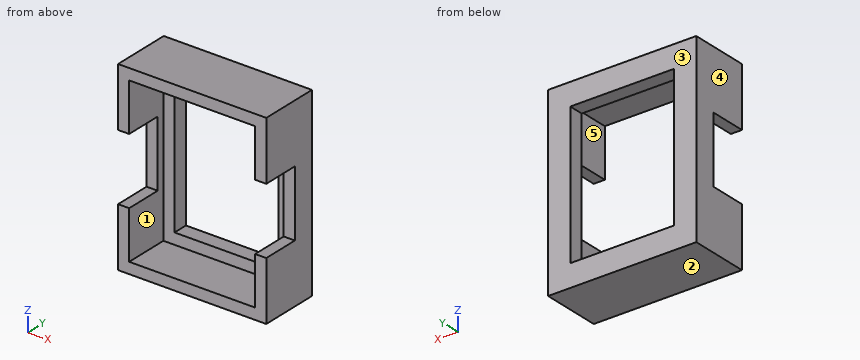
from build123d import *

# Parameters (mm, degrees)
SKETCH1_W           = 20
SKETCH1_H           = 25
BOSS_EXTRUDE1_DEPTH = 8
SKETCH2_W           = 9
SKETCH2_H           = 5
CUT_EXTRUDE1_DEPTH  = 31
SKETCH3_W           = 17
SKETCH3_H           = 22
CUT_EXTRUDE2_DEPTH  = 6
SKETCH4_W           = 14
SKETCH4_H           = 19
CUT_EXTRUDE3_DEPTH  = 7


with BuildPart() as part:
    # Sketch1 → Boss-Extrude1 (new body)
    with BuildSketch(Plane(origin=(0, 0, 0), x_dir=(1, 0, 0), z_dir=(0, 1, 0))):
        with Locations((-10.903225806, -2.629032258)):
            Rectangle(SKETCH1_W, SKETCH1_H)
    extrude(amount=BOSS_EXTRUDE1_DEPTH)

    # Sketch2 → Cut-Extrude1 (cut)
    with BuildSketch(Plane.ZY.offset(20.903225806)):
        with Locations((2.629032258, 2.5)):
            Rectangle(SKETCH2_W, SKETCH2_H)
    extrude(amount=-CUT_EXTRUDE1_DEPTH, mode=Mode.SUBTRACT)

    # Sketch3 → Cut-Extrude2 (cut)
    with BuildSketch(Plane.XZ):
        with Locations((-10.903225806, 2.629032258)):
            Rectangle(SKETCH3_W, SKETCH3_H)
    extrude(amount=-CUT_EXTRUDE2_DEPTH, mode=Mode.SUBTRACT)

    # Sketch4 → Cut-Extrude3 (cut)
    with BuildSketch(Plane(origin=(0, 8, 0), x_dir=(1, 0, 0), z_dir=(0, 1, 0))):
        with Locations((-10.903225806, -2.629032258)):
            Rectangle(SKETCH4_W, SKETCH4_H)
    extrude(amount=-CUT_EXTRUDE3_DEPTH, mode=Mode.SUBTRACT)


solid = part.part
Geometry check sheet. Reference: the model listing, model coordinates, mm. Face numbers are marked on the shaded views. A direction names the side the tool comes from. Coordinates: 2 decimals unless noted, no trailing zeros. Order: outer loops, then holes, each group sorted by start corner. A loop starts at its lowest first (then second) coordinate and runs counter-clockwise, first axis right, second up. Notation, with made-up numbers: (54.5, -24) - (88.5, -24) arc R21 cw to (88.5, 2) - close; hole circle Ø6 at (13, 10). An arc over 180 degrees is marked (long way). One line per item, written item: value.
(1) Sectioned sample at C-C (x = -8.75). Enter the section's corners in (y, z).
Data:
outline: (0, -9.87) - (8, -9.87) - (8, -6.87) - (6, -6.87) - (6, -8.37) - (0, -8.37) - close; (0, 13.63) - (6, 13.63) - (6, 12.13) - (8, 12.13) - (8, 15.13) - (0, 15.13) - close
(2) Depth check by flat-ended pin: pin 1 Ø0.5 at (x, z) = (-2, 1.5) entering from -Y. Enter the tip coordinate at first touch or a pass-through.
Data:
pin 1: stops at y = 5
(3) Release check for a two-part mould opening along X. For the marked faces 3, 4 and 5 record: +X half, -X half, draft (parallel to the pull), parting line (faces both ways), or undercut.
Data:
face 3: draft
face 4: -X half
face 5: undercut
(4) Sectioned sample at B-B (y = 4.25). Enter the section's corners in (x, z).
Data:
outline: (-20.9, -9.87) - (-0.9, -9.87) - (-0.9, -1.87) - (-2.4, -1.87) - (-2.4, -8.37) - (-19.4, -8.37) - (-19.4, -1.87) - (-20.9, -1.87) - close; (-20.9, 7.13) - (-19.4, 7.13) - (-19.4, 13.63) - (-2.4, 13.63) - (-2.4, 7.13) - (-0.9, 7.13) - (-0.9, 15.13) - (-20.9, 15.13) - close
(5) Thickness scan on probe 1 along X at (y, z) = (1.75, -2.25); probe 2 along Z at (x, y) = (-7.5, 6.5); probe 3 along X at (y, z) = (7.5, 8.25). Record the ranges inside material, lowest first. Write a range as from..to.
Data:
probe 1: x = -20.9..-19.4, -2.4..-0.9
probe 2: z = -9.87..-6.87, 12.13..15.13
probe 3: x = -20.9..-17.9, -3.9..-0.9
(6) Access from +Z, -Z, +X, -X, +Y, -Y to the whole of each face (thin tool, end or side, straight path). Record for the marked faces 1 and 2.
Data:
face 1: -Y
face 2: -Z, +X, -X, +Y, -Y
(7) Sectioned sample at A-A (z = 4.5). Enter the section's corners in (x, y).
Data:
outline: (-20.9, 5) - (-19.4, 5) - (-19.4, 6) - (-17.9, 6) - (-17.9, 8) - (-20.9, 8) - close; (-3.9, 6) - (-2.4, 6) - (-2.4, 5) - (-0.9, 5) - (-0.9, 8) - (-3.9, 8) - close
(8) Sectioned sample at D-D (y = 7.5). Enter the section's corners in (x, z).
Data:
outline: (-20.9, -9.87) - (-0.9, -9.87) - (-0.9, 15.13) - (-20.9, 15.13) - close; hole (-17.9, -6.87) - (-3.9, -6.87) - (-3.9, 12.13) - (-17.9, 12.13) - close
